from build123d import *

# Parameters (mm, degrees)
SKETCH2_R           = 2.5
BOSS_EXTRUDE1_DEPTH = 3


with BuildPart() as part:
    # Sketch2 → Boss-Extrude1 (new body)
    with BuildSketch(Plane.XY):
        with BuildLine():
            Line((16.770370099, 3.355657737), (46.770370099, 3.355657737))
            ThreePointArc((46.770370099, 3.355657737), (49.270370099, 0.855657737), (46.770370099, -1.644342263))
            Line((46.770370099, -1.644342263), (23.033866759, -1.644342263))
            ThreePointArc((23.033866759, -1.644342263), (22.849090853, -1.767805576), (22.892445403, -1.985763619))
            Line((22.892445403, -1.985763619), (24.904577438, -3.997895654))
            ThreePointArc((24.904577438, -3.997895654), (25.066789112, -4.106282029), (25.258130828, -4.144342263))
            Line((25.258130828, -4.144342263), (46.770370099, -4.144342263))
            ThreePointArc((46.770370099, -4.144342263), (51.770370099, 0.855657737), (46.770370099, 5.855657737))
            Line((46.770370099, 5.855657737), (1.770370099, 5.855657737))
            ThreePointArc((1.770370099, 5.855657737), (-3.229629901, 0.855657737), (1.770370099, -4.144342263))
            Line((1.770370099, -4.144342263), (17.75199348, -4.144342263))
            ThreePointArc((17.75199348, -4.144342263), (17.936769387, -4.020878949), (17.893414837, -3.802920907))
            Line((17.893414837, -3.802920907), (15.002603146, -0.912109216))
            ThreePointArc((15.002603146, -0.912109216), (14.460671268, 1.812366318), (16.770370099, 3.355657737))
        make_face()
        with Locations((7.770370099, 0.855657737)):
            Circle(SKETCH2_R, mode=Mode.SUBTRACT)
    extrude(amount=BOSS_EXTRUDE1_DEPTH)


solid = part.part
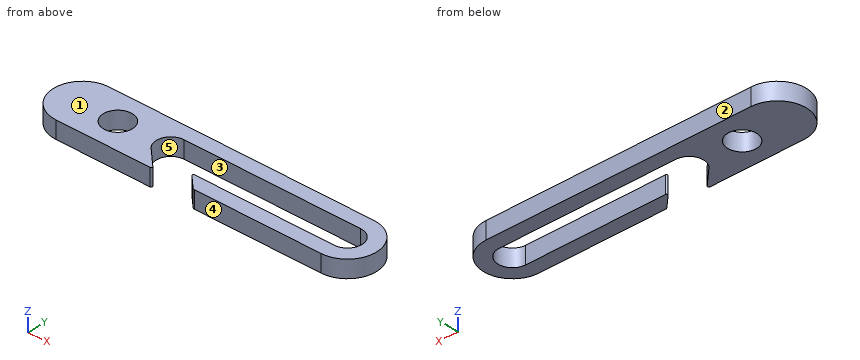
Could you check a few things on this model? Use its own coordinates, in mm. Face numbers are marked on the shaded views. A direction names the side the tool comes from. Give positions to 0.01 mm unless a question says otherwise; leave off trailing zeros. Order: outer loops, then holes, each group sorted by start corner. A loop starts at its lowest first (then second) coordinate and runs counter-clockwise, first axis right, second up.
Item 1: If we section it at A-A, the plane x = 30: Write out the boundary of the cut face in (y, z).
Item 2: I need wall thicknesses on line 1 (X direction, y = 1, z = 2.35); line 2 (X direction, y = 1.75, z = 0.75); line 3 (Y direction, x = 35.5, z = 2.45). Which ranges of each line are inside material? Lowest first, please.
Item 3: If we mould it in two halves opening along Y, with no side actions, what happens to the marked faces 1, 2 and 3? For each: pulls with the +Y half, pulls with the -Y half, needs draft (parallel to the pull), parting line crosses it, or undercut.
Item 4: If we section it at D-D, the plane y = -2.5: Write out the boundary of the cut face in (x, z), plus the area to 3 significant figures.
Item 5: I'm going to push a flat-ended pin straight in: pin 1 (3 mm diameter, centred on x = 7.77, y = 0.86, fed in from +Z). Where does the tip first touch, or does it pass through?
Item 6: If we section it at C-C, the plane z = 1.3: Write out the boundary of the cut face in (x, y).
Item 7: If we section it at B-B, the plane y = 1.5: Write out the boundary of the cut face in (x, z).
Item 8: For the marked faces 4 and 5, which set-ups out of +Z, -Z, +X, -X, +Y, -Y let a thin tool reach every point of the face, with its end or its side?
Values:
1. outline: (-4.14, 0) - (-1.64, 0) - (-1.64, 3) - (-4.14, 3) - close; (3.36, 0) - (5.86, 0) - (5.86, 3) - (3.36, 3) - close
2. line 1: x = -3.23 to 5.27, 10.27 to 14.27, 49.27 to 51.77
2. line 2: x = -3.15 to 5.44, 10.1 to 14.44, 49.1 to 51.69
2. line 3: y = -4.14 to -1.64, 3.36 to 5.86
3. face 1: needs draft
3. face 2: pulls with the +Y half
3. face 3: undercut
4. outline: (-1.94, 0) - (16.59, 0) - (16.59, 3) - (-1.94, 3) - close; (23.41, 0) - (50.48, 0) - (50.48, 3) - (23.41, 3) - close
4. area: 137 mm2
5. pin 1: passes through
6. outline: (1.77, -4.14) - (17.75, -4.14) arc R0.2 ccw to (17.89, -3.8) - (15, -0.91) arc R2.5 cw to (16.77, 3.36) - (46.77, 3.36) arc R2.5 cw to (46.77, -1.64) - (23.03, -1.64) arc R0.2 ccw to (22.89, -1.99) - (24.9, -4) arc R0.5 ccw to (25.26, -4.14) - (46.77, -4.14) arc R5 ccw to (46.77, 5.86) - (1.77, 5.86) arc R5 ccw to start; hole circle Ø5 at (7.77, 0.86)
7. outline: (-3.19, 0) - (5.35, 0) - (5.35, 3) - (-3.19, 3) - close; (10.19, 0) - (14.35, 0) - (14.35, 3) - (10.19, 3) - close; (49.19, 0) - (51.73, 0) - (51.73, 3) - (49.19, 3) - close
8. face 4: +Z, -Z, +X, -X, -Y
8. face 5: +Z, -Z
